```python
from build123d import *

# Parameters (mm, degrees)
SKETCH_1_W      = 40
SKETCH_1_H      = 10
EXTRUDE_1_DEPTH = 2.5
SKETCH_3_W      = 4
SKETCH_3_H      = 10
EXTRUDE_3_DEPTH = 3
SKETCH_4_W      = 15
SKETCH_4_H      = 1.5
SKETCH_4_W_2    = 3
SKETCH_4_H_2    = 3.5
EXTRUDE_4_DEPTH = 3
CHAMFER_1_SIZE  = 1.5
SKETCH_6_R      = 3
SKETCH_6_R_2    = 1.6
EXTRUDE_5_DEPTH = 5.5
SKETCH_7_W      = 2.5
SKETCH_7_H      = 10
EXTRUDE_6_DEPTH = 10
SKETCH_8_W      = 4
SKETCH_8_H      = 1.5
EXTRUDE_7_DEPTH = 5.5
SKETCH_9_W      = 33
SKETCH_9_H      = 10
EXTRUDE_8_DEPTH = 3
CHAMFER_2_SIZE  = 3


with BuildPart() as part:
    # 草图1 → 凸台-拉伸1 (new body)
    with BuildSketch(Plane.XY):
        with Locations((20, 5)):
            Rectangle(SKETCH_1_W, SKETCH_1_H)
    extrude(amount=EXTRUDE_1_DEPTH)

    # 草图3 → 凸台-拉伸3 (add)
    with BuildSketch(Plane(origin=(0, 0, 0), x_dir=(-1, 0, 0), z_dir=(0, 0, -1))):
        with Locations((-38, 5)):
            Rectangle(SKETCH_3_W, SKETCH_3_H)
    extrude(amount=EXTRUDE_3_DEPTH)

    # 草图4 → 凸台-拉伸4 (add)
    with BuildSketch(Plane(origin=(0, 0, 0), x_dir=(-1, 0, 0), z_dir=(0, 0, -1))):
        with Locations((-28.5, 5.75)):
            Rectangle(SKETCH_4_W, SKETCH_4_H)
        with Locations((-28.5, 4.25)):
            Rectangle(SKETCH_4_W, SKETCH_4_H)
        with Locations((-19.5, 5.75)):
            Rectangle(SKETCH_4_W_2, SKETCH_4_H)
        with Locations((-19.5, 4.25)):
            Rectangle(SKETCH_4_W_2, SKETCH_4_H)
        with Locations((-19.5, 8.25)):
            Rectangle(SKETCH_4_W_2, SKETCH_4_H_2)
        with Locations((-19.5, 1.75)):
            Rectangle(SKETCH_4_W_2, SKETCH_4_H_2)
        with Locations((-10.5, 5.75)):
            Rectangle(SKETCH_4_W, SKETCH_4_H)
        with Locations((-10.5, 4.25)):
            Rectangle(SKETCH_4_W, SKETCH_4_H)
        with Locations((-1.5, 5.75)):
            Rectangle(SKETCH_4_W_2, SKETCH_4_H)
        with Locations((-1.5, 4.25)):
            Rectangle(SKETCH_4_W_2, SKETCH_4_H)
        with Locations((-1.5, 8.25)):
            Rectangle(SKETCH_4_W_2, SKETCH_4_H_2)
        with Locations((-1.5, 1.75)):
            Rectangle(SKETCH_4_W_2, SKETCH_4_H_2)
    extrude(amount=EXTRUDE_4_DEPTH)

    # 倒角1
    chamfer_1_edges = [part.edges().sort_by_distance(p)[0] for p in [
        (10.5, 3.5, 0),
        (28.5, 3.5, 0),
    ]]
    chamfer(chamfer_1_edges, length=CHAMFER_1_SIZE)
    chamfer_1_2_edges = [part.edges().sort_by_distance(p)[0] for p in [
        (10.5, 3.5, -3),
        (28.5, 3.5, -3),
    ]]
    chamfer(chamfer_1_2_edges, length=CHAMFER_1_SIZE - 0.0001)  # a hair under: the kernel refuses the full size

    # 草图6 → 凸台-拉伸5 (add)
    with BuildSketch(Plane.XY.offset(2.5)):
        with Locations(Location((20, 5, 0), (0, 0, 180))):
            Circle(SKETCH_6_R)
        with Locations((20, 5)):
            Circle(SKETCH_6_R_2, mode=Mode.SUBTRACT)
    extrude(amount=EXTRUDE_5_DEPTH)

    # 草图7 → 凸台-拉伸6 (add)
    with BuildSketch(Plane.ZY):
        with Locations((1.25, 5)):
            Rectangle(SKETCH_7_W, SKETCH_7_H)
    extrude(amount=EXTRUDE_6_DEPTH)

    # 草图8 → 凸台-拉伸7 (add)
    with BuildSketch(Plane.XY.offset(2.5)):
        with Locations((15.09526249, 5)):
            Rectangle(SKETCH_8_W, SKETCH_8_H)
        with Locations((24.90473751, 5)):
            Rectangle(SKETCH_8_W, SKETCH_8_H)
    extrude(amount=EXTRUDE_7_DEPTH)

    # 草图9 → 凸台-拉伸8 (add)
    with BuildSketch(Plane(origin=(0, 0, 0), x_dir=(-1, 0, 0), z_dir=(0, 0, -1))):
        with Locations((-19.5, 5)):
            Rectangle(SKETCH_9_W, SKETCH_9_H)
    extrude(amount=EXTRUDE_8_DEPTH)

    # 倒角2
    chamfer_2_edges = [part.edges().sort_by_distance(p)[0] for p in [
        (0, 5, -3),
    ]]
    chamfer(chamfer_2_edges, length=CHAMFER_2_SIZE - 0.0001)  # a hair under: the kernel refuses the full size


solid = part.part
```
Can you work these out from the model? Positions are in its coordinate system, mm. A direction names the side the tool comes from. Coordinates: 2 decimals unless noted, no trailing zeros. Loops run counter-clockwise (first coordinate to the right, second up) from the corner with the lowest first, then second, coordinate; pieces in that order, holes last.
Item 1: Suppose I cut it at D-D (x = 20). Please give me the cut outline in (y, z), then the cut area to 3 significant figures.
Answers below:
outline: (0, -3) - (10, -3) - (10, 2.5) - (8, 2.5) - (8, 8) - (6.6, 8) - (6.6, 2.5) - (3.4, 2.5) - (3.4, 8) - (2, 8) - (2, 2.5) - (0, 2.5) - close
area: 70.4 mm2
Item 2: Suppose I cut it at B-B (x = 14). Please give me the cut outline in (y, z).
Answers below:
outline: (0, -3) - (10, -3) - (10, 2.5) - (5.75, 2.5) - (5.75, 8) - (4.25, 8) - (4.25, 2.5) - (0, 2.5) - close
Item 3: Which directions (+Z, -Z, +X, -X, +Y, -Y) give clear straight access to the entire face, cutting with the end or side of a thin tool? Please do faces 4 (the face through (15, 5.75, 5)), 5 (the face through (25, 5.75, 5)), 6 (the face through (13.095, 5, 5)), 7 (the face through (26.905, 5, 5)).
Answers below:
face 4: +Z, -X, +Y
face 5: +Z, +X, +Y
face 6: +Z, -X, +Y, -Y
face 7: +Z, +X, +Y, -Y
Item 4: Please list where these lines run through material, in increasing order: L1, parallel to Y at x = 20, z = 6.2; L2, parallel to Z at x = 16, y = 3.5; L3, parallel to Z at x = -3, y = 3.25.
Answers below:
L1: y = 2 to 3.4, 6.6 to 8
L2: z = -3 to 2.5
L3: z = 0 to 2.5
Item 5: If we mould it in two halves opening along X, with no side actions, what happens to faces 1 (the face through (15, 4.25, 5)), 2 (the face through (20, 2, 5)), 3 (the face through (18.73, 4.03, 5.21))? For each: released by +X, released by -X, zero draft, split by the parting line, or undercut.
Answers below:
face 1: zero draft
face 2: split by the parting line
face 3: undercut
Item 6: I'm going to push flat-ended pins straight in: pin 1 (5 mm diameter, centred on y = 8, z = 5.5, fed in from +X); pin 2 (2 mm diameter, centred on x = 1, y = 7.5, fed in from -Z); pin 3 (1 mm diameter, centred on x = 20, y = 5.5, fed in from +Z). Where does each tip first touch, or does it pass through?
Answers below:
pin 1: stops at x = 26.9
pin 2: stops at z = -2
pin 3: stops at z = 2.5
